Source: three-view drawing plus pictorial views. Frame: mm from the lowest corner of the part. Coordinates: 2 decimals unless noted, no trailing zeros. Order: outer loops, then holes, each group sorted by start corner. A loop starts at its lowest first (then second) coordinate and runs counter-clockwise, first axis right, second up. Notation, with made-up numbers: (67, -27) - (96, -27) arc R35 cw to (96, 9) - close; hole circle Ø3 at (87, 60). An arc over 180 degrees is marked (long way). Use a Markdown table: item, result. Add a question column.
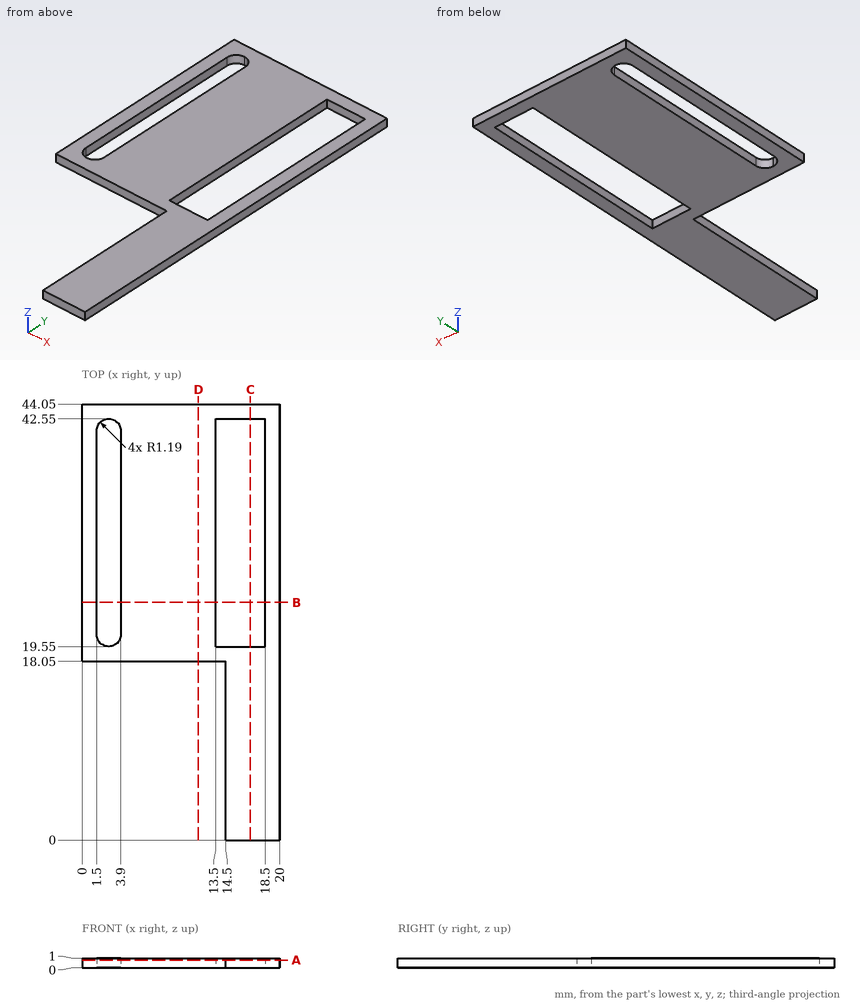
1) Section B-B (y = 24). Return loops of the section in (x, z), then the cut area to 3 significant figures.
2) Section A-A (z = 0.8). Give the number of separate pieces and of enclosed holes in the cut face, then the cut area to 3 significant figures.
3) Pin query (flat end, axial travel): pin 1 (8 mm diameter, centred on x = 15, y = 36.5, fed in from +Z). Return the tip coordinate at first contact, or that it passes through.
4) Section C-C (x = 17). Return loops of the section in (y, z), then the cut area to 4 significant figures.
5) Ray query, line 1 along X through (y, z) = (34.5, 0.65); line 2 along Y through (x, z) = (15.25, 0.1); line 3 along Y through (x, z) = (11, 0.95). Return the intervals inside material, ascending.
6) Section D-D (x = 11.75). Return loops of the section in (y, z).
Values follow:
| question | item | result |
|---|---|---|
| 1 | outline | (0, 0) - (1.5, 0) - (1.5, 1) - (0, 1) - close; (3.9, 0) - (13.5, 0) - (13.5, 1) - (3.9, 1) - close; (18.5, 0) - (20, 0) - (20, 1) - (18.5, 1) - close |
| 1 | area | 12.6 mm² |
| 2 | separate pieces | 1 |
| 2 | enclosed holes | 2 |
| 2 | area | 450 mm² |
| 3 | pin 1 | stops at z = 1 |
| 4 | outline | (0, 0) - (19.55, 0) - (19.55, 1) - (0, 1) - close; (42.55, 0) - (44.05, 0) - (44.05, 1) - (42.55, 1) - close |
| 4 | area | 21.05 mm² |
| 5 | line 1 | x = 0 to 1.5, 3.9 to 13.5, 18.5 to 20 |
| 5 | line 2 | y = 0 to 19.55, 42.55 to 44.05 |
| 5 | line 3 | y = 18.05 to 44.05 |
| 6 | outline | (18.05, 0) - (44.05, 0) - (44.05, 1) - (18.05, 1) - close |
